The listing builds one solid part. Answer for the finished solid, in the listing's coordinates (mm). Face numbers are marked on the shaded views. Coordinates: 2 decimals unless noted, no trailing zeros. Order: outer loops, then holes, each group sorted by start corner. A loop starts at its lowest first (then second) coordinate and runs counter-clockwise, first axis right, second up.
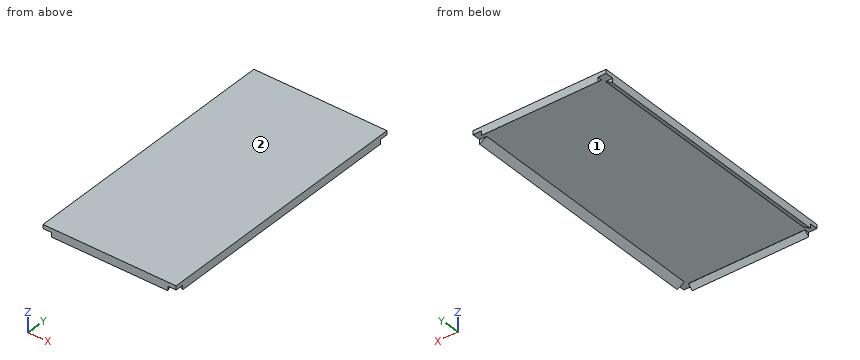
```python
from build123d import *

# Parameters (mm, degrees)
F1_DEPTH = 203.2
F3_DEPTH = 44.45
F5_DEPTH = 6.35
F7_DEPTH = 6.35


# Not quite as in the source:
# - a pattern or mirror of a feature is missing from the dataset's text; its kind, count and spacing are read off the source's solid


with BuildPart() as f1:
    # F0 (on Front) → F1 (new body)
    with BuildSketch(Plane.XZ):
        Polygon((50.8, 0), (0, 0), (-50.8, 0), (-50.8, -6.35), (-45.386130618, -3.0314885393), (45.382719487, -3.0314885393), (50.8, -6.35), align=None)
    extrude(amount=F1_DEPTH)

    # F2 (on Right) → F3 (join, symmetric)
    with BuildSketch(Plane.YZ):
        Polygon((0, -6.3831382431), (0, 0), (-3.5511243623, 0), (-3.5511243623, -3.1539145857), align=None)
    f3 = extrude(amount=F3_DEPTH, both=True)

    # F3_copies: F3 across plane
    add(f3.mirror(Plane(origin=(0, -101.6, 0), x_dir=(0, 0, -1), z_dir=(0, -1, 0))))

    # F4 (on Front) → F5 (cut)
    with BuildSketch(Plane.XZ):
        Polygon((50.8, -3.0314885393), (45.382719487, -3.0314885393), (50.8, -6.35), align=None)
        Polygon((-50.8, -3.0314885393), (-50.8, -6.35), (-45.382719487, -3.0314885393), align=None)
    extrude(amount=F5_DEPTH, mode=Mode.SUBTRACT)

    # F6 (on face) → F7 (cut)
    with BuildSketch(Plane.XZ.offset(203.2)):
        Polygon((-50.8, -6.35), (-45.386130618, -3.0314885393), (-50.8, -3.0314885393), align=None)
        Polygon((50.8, -6.35), (50.8, -3.0314885393), (45.382719487, -3.0314885393), align=None)
    extrude(amount=-F7_DEPTH, mode=Mode.SUBTRACT)


solid = f1.part
```
1) A cutting plane is placed at B-B, the plane y = -13. Write down the section's boundary in (x, z).
2) Straight lines are drawn through the part: probe 1 along Z at (x, y) = (-15, -155.5); probe 2 along X at (y, z) = (-150.5, -3.75); probe 3 along Y at (x, z) = (-8, -3.25). For each, find the intervals that lie inside material, in ascending order.
3) The mould has two halves that part along Y. Classify the marked faces 1 and 2: released by +Y, released by -Y, zero draft, split by the parting line, or undercut.
4) Each of these flat-tipped pins is pushed along its axis until it touches: P1, Ø1.7, axis at x = -48, z = -5.5, coming from the -Y side; P2, Ø1, axis at x = -48.5, z = -4.5, coming from the +Y side; P3, Ø4, axis at x = -5.5, y = -101, coming from the -Z side; P4, Ø2.5, axis at y = -201.5, z = -4, coming from the +X side. Where does it stop, or does it pass through?
5) A cutting plane is placed at A-A, the plane x = 27.5. Write down the section's boundary in (y, z), plus the area to 3 significant figures.
Working result:
1. outline: (-50.8, -6.35) - (-45.39, -3.03) - (45.38, -3.03) - (50.8, -6.35) - (50.8, 0) - (-50.8, 0) - close
2. probe 1: z = -3.03 to 0
2. probe 2: x = -50.8 to -46.56, 46.56 to 50.8
2. probe 3: y = -203.2 to -199.75, -3.45 to 0
3. face 1: undercut
3. face 2: zero draft
4. P1: stops at y = -196.85
4. P2: stops at y = -6.35
4. P3: stops at z = -3.03
4. P4: stops at x = 50.8
5. outline: (-203.2, -6.38) - (-199.65, -3.15) - (-199.65, -3.03) - (-3.55, -3.03) - (-3.55, -3.15) - (0, -6.38) - (0, 0) - (-203.2, 0) - close
5. area: 628 mm2
